from build123d import *

# Parameters (mm, degrees)
F0_R     = 21.5
F1_DEPTH = 30
F2_SIZE2 = 25
F2_SIZE  = 11.5
F3_DEPTH = 30
F4_R     = 21.5
F5_DEPTH = 43


# Not quite as in the source:
# - a fillet or chamfer that OpenCascade refuses, or shapes differently, is made with other operations: its cross-section is extruded or revolved along the edge and cut away or added


with BuildPart() as f1:
    # F0 (on Top) → F1 (new body)
    with BuildSketch(Plane.XY):
        Circle(F0_R)
    extrude(amount=F1_DEPTH)

    # F2
    f2_edges = [f1.edges().sort_by_distance(p)[0] for p in [
        (-21.5, 0, 30),
    ]]
    f2_side = f1.faces().sort_by_distance((0, 0, 30))[0]
    chamfer(f2_edges, length=F2_SIZE, length2=F2_SIZE2, reference=f2_side)

    # F3 (add): a face of the model
    f3_faces = [f1.faces().sort_by_distance(p)[0] for p in [
        (0, 0, 30),
    ]]
    extrude(f3_faces, amount=F3_DEPTH)

    # F4 (on face) → F5 (join)
    with BuildSketch(Plane.XY.offset(60)):
        Circle(F4_R)
    extrude(amount=F5_DEPTH)

    # F6: fillet of radius 21.499 on 2 edges, made by hand

    # F6_s1 → F6_t2 (revolve, cut)
    with BuildSketch(Plane.XZ):
        with BuildLine():
            ThreePointArc((21.5, 81.501), (15.2030886887, 96.7030886887), (0.001, 103))
            Line((0.001, 103), (21.5, 103))
            Line((21.5, 103), (21.5, 81.501))
        make_face()
    revolve(axis=Axis((0, 0, 103), (0, 0, 1)), mode=Mode.SUBTRACT)

    # F6_s3 → F6_t4 (revolve, cut)
    with BuildSketch(Plane.XZ):
        with BuildLine():
            ThreePointArc((21.5, 79.0322620831), (18.4017540878, 67.913842681), (10, 60))
            Line((10, 60), (21.5, 60))
            Line((21.5, 60), (21.5, 79.0322620831))
        make_face()
    revolve(axis=Axis((0, 0, 60), (0, 0, 1)), mode=Mode.SUBTRACT)


solid = f1.part
Geometry: final body of the model. Coordinates: model frame, mm. A direction names the side the tool comes from. Round coordinates to 2 decimals unless told otherwise and drop trailing zeros. Loops run counter-clockwise (first coordinate to the right, second up) from the corner with the lowest first, then second, coordinate; pieces in that order, holes last. Notation, with made-up numbers: (50, 48) -> (97, 48) arc R19 cw to (97, 55) -> close; hole circle Ø2 at (-11, 53). An arc over 180 degrees is marked (long way). One line per question, with ' | ' between items. Start each with the question number.
1. Section B-B on z = 22.5. Output: boundary loops of the cut face in (x, y), and give its area (3 significant figures).
2. Section A-A on z = 49.5. Output: boundary loops of the cut face in (x, y), and give its area (3 significant figures).
3. Set-up query: faces 1 (the face through (-2.17, -9.76, 44.79)), 2 (the face through (0, 0, 0)). Return all of +Z, -Z, +X, -X, +Y, -Y with unobstructed straight access to the full face (end or side cutting, diameter ignored); none if empty.
4. Line query: line 1 along Z through (x, y) = (-8.5, 11.5); line 2 along Z through (x, y) = (-14.5, -10.5); line 3 along Y through (x, z) = (7, 53). Output: solid intervals per line, ascending. Write a range as [from, to].
5. Contact query for flat-ended pins moving along their axis: pin 1 (10 mm diameter, centred on y = -15, z = 87.5, fed in from +X); pin 2 (6 mm diameter, centred on y = 5, z = 21, fed in from +X); pin 3 (4 mm diameter, centred on y = -16.5, z = 84, fed in from +X). Output: stop coordinate, or through.
Returned:
1) outline: circle Ø26.9 at (0, 0) | area: 568 mm2
2) outline: circle Ø20 at (0, 0) | area: 314 mm2
3) face 1: none | face 2: -Z, +X, -X, +Y, -Y
4) line 1: z = [0, 20.65], [62.98, 97.56] | line 2: z = [0, 12.82], [67.13, 93.41] | line 3: y = [-7.14, 7.14]
5) pin 1: stops at x = 18.38 | pin 2: stops at x = 14.93 | pin 3: stops at x = 15.7
